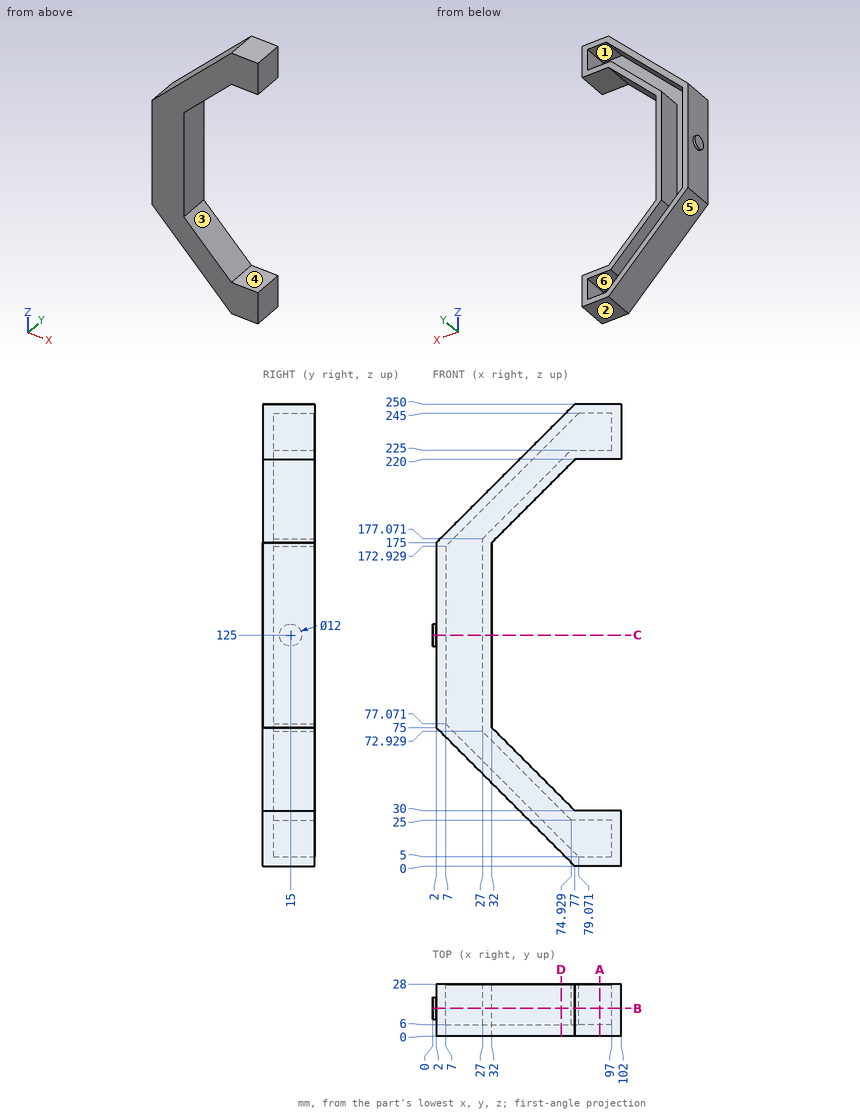
Print and shaded views of the part. All mm, measured from the part's lowest x, y and z. A direction names the side the tool comes from. Round coordinates to 2 decimals unless told otherwise and drop trailing zeros. Write each loop counter-clockwise with the first axis right and the second up, starting at its lowest first coordinate (ties: lowest second). Pieces come first, ordered by that corner, then holes. Notation, with made-up numbers: M 61,-6 L 93,-6 A19 ccw 93,21 Z; hole C 27,9 d8. An arc over 180 degrees is marked long. Use a Markdown table: item, result. Add a question column.
1. Flat gauge pins, fed straight in: P1, Ø6, axis at x = 37, z = 166.5, coming from the +Y side; P2, Ø10, axis at y = 15.5, z = 19.5, coming from the -X side; P3, Ø2, axis at x = 26, y = 13, coming from the +Z side; P4, Ø1.5, axis at x = 41.5, y = 17.5, coming from the -Z side. Where does each tip first touch, or does it go through?
2. Pull direction X, two halves, no side cores. Call the marked faces 1, 2 and 3: released by +X, released by -X, zero draft, split by the parting line, or undercut.
3. Slice it at B-B on y = 15. Give the cut face in (x, z).
4. 3-axis set-ups, long thin cutter, end or side, ignore diameter. For the marked faces 4, 5 and 6: which of +Z, -Z, +X, -X, +Y, -Y reach the whole face in a straight line?
5. Slice it at D-D on x = 69.5. Give the cut face in (y, z), then the cut area to 3 significant figures.
6. Slice it at A-A on x = 90.5. Give the cut face in (y, z), then the cut area to 3 significant figures.
7. Slice it at C-C on z = 125. Give the cut face in (x, y).
8. Drill centre lines: probe 1 along Z at (x, y) = (87, 12); probe 2 along Z at (x, y) = (88.5, 5.75); probe 3 along X at (y, z) = (9, 124). Where is each one in solid material? Low to high.
Reply:
| question | item | result |
|---|---|---|
| 1 | P1 | passes through |
| 1 | P2 | stops at x = 52.5 |
| 1 | P3 | stops at z = 200 |
| 1 | P4 | stops at z = 34.75 |
| 2 | face 1 | undercut |
| 2 | face 2 | zero draft |
| 2 | face 3 | released by +X |
| 3 | outline | M 0,119 L 2,119 L 2,75 L 77,0 L 102,0 L 102,30 L 77,30 L 32,75 L 32,175 L 77,220 L 102,220 L 102,250 L 77,250 L 2,175 L 2,131 L 0,131 Z; hole M 7,77.07 L 79.07,5 L 97,5 L 97,25 L 74.93,25 L 27,72.93 L 27,177.07 L 74.93,225 L 97,225 L 97,245 L 79.07,245 L 7,172.93 Z |
| 4 | face 4 | +X, +Y, -Y |
| 4 | face 5 | -Z, -X, +Y, -Y |
| 4 | face 6 | +Y |
| 5 | outline | M 0,7.5 L 28,7.5 L 28,14.57 L 6,14.57 L 6,30.43 L 28,30.43 L 28,37.5 L 0,37.5 Z; M 0,212.5 L 28,212.5 L 28,219.57 L 6,219.57 L 6,235.43 L 28,235.43 L 28,242.5 L 0,242.5 Z |
| 5 | area | 982 mm^2 |
| 6 | outline | M 0,0 L 28,0 L 28,5 L 6,5 L 6,25 L 28,25 L 28,30 L 0,30 Z; M 0,220 L 28,220 L 28,225 L 6,225 L 6,245 L 28,245 L 28,250 L 0,250 Z |
| 6 | area | 800 mm^2 |
| 7 | outline | M 0,9 L 2,9 L 2,0 L 32,0 L 32,28 L 27,28 L 27,6 L 7,6 L 7,28 L 2,28 L 2,21 L 0,21 Z |
| 8 | probe 1 | z = 0 to 5, 25 to 30, 220 to 225, 245 to 250 |
| 8 | probe 2 | z = 0 to 30, 220 to 250 |
| 8 | probe 3 | x = 2 to 7, 27 to 32 |
